Design review of the part built by this model. Coordinates are the model's own, in mm. Face numbers are marked on the shaded views. A direction names the side the tool comes from. Coordinates: 2 decimals unless noted, no trailing zeros. Loops run counter-clockwise (first coordinate to the right, second up) from the corner with the lowest first, then second, coordinate; pieces in that order, holes last. Notation, with made-up numbers: M -40,-8 L 11,-8 A22 cw 11,31 Z; hole C -32.75,82.5 d3. An arc over 180 degrees is marked long. One line per item, written item: value.
```python
from build123d import *

# Parameters (mm, degrees)
F0_W     = 165
F0_H     = 40
F1_DEPTH = 10
F2_SIZE2 = 9.99999
F2_SIZE  = 4.99999
F3_SIZE2 = 4.99999
F3_SIZE  = 9.99999
F4_W     = 44
F4_H     = 4
F5_DEPTH = 18
F4_H_2   = 9
F6_DEPTH = 8


# Not quite as in the source:
# - a fillet or chamfer is up to 0.001 mm smaller than in the source, because OpenCascade refuses the exact size


with BuildPart() as f1:
    # F0 (on Top) → F1 (new body)
    with BuildSketch(Plane.XY):
        with Locations((82.5, 20)):
            Rectangle(F0_W, F0_H)
    extrude(amount=F1_DEPTH)

    # F2 (size 5 and 10 in the source; OpenCascade refuses exactly that, so slightly less here)
    f2_edges = [f1.edges().sort_by_distance(p)[0] for p in [
        (165, 20, 10),
    ]]
    f2_side = f1.faces().sort_by_distance((82.5, 20, 10))[0]
    chamfer(f2_edges, length=F2_SIZE, length2=F2_SIZE2, reference=f2_side)

    # F3 (size 10 and 5 in the source; OpenCascade refuses exactly that, so slightly less here)
    f3_edges = [f1.edges().sort_by_distance(p)[0] for p in [
        (0, 20, 10),
    ]]
    f3_side = f1.faces().sort_by_distance((0, 20, 5))[0]
    chamfer(f3_edges, length=F3_SIZE, length2=F3_SIZE2, reference=f3_side)

    # F4 (on face) → F5 (join)
    with BuildSketch(Plane.XY.offset(10)):
        with Locations((135, 30.5)):
            Rectangle(F4_W, F4_H)
        with Locations((135, 9.5)):
            Rectangle(F4_W, F4_H)
    extrude(amount=F5_DEPTH)

    # F4 (on face) → F6 (join)
    with BuildSketch(Plane.XY.offset(10)):
        with Locations((135, 20)):
            Rectangle(F4_W, F4_H_2)
    extrude(amount=F6_DEPTH)


solid = f1.part
```
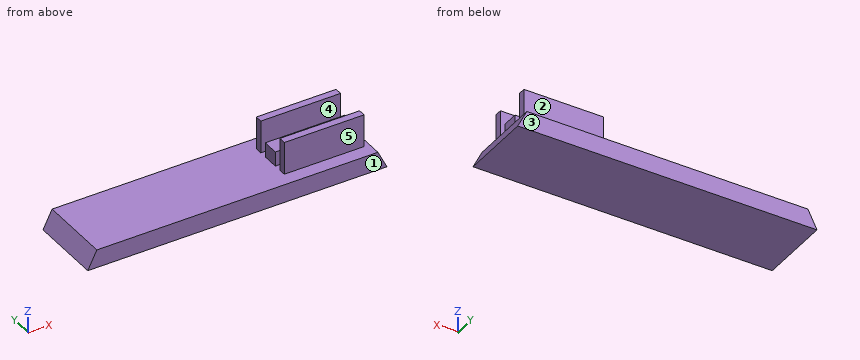
(1) Tool access review of the marked faces 1 and 2: name each direction out of +Z, -Z, +X, -X, +Y, -Y from which nothing blocks a thin tool from reaching the whole face with its end or side.
Reply:
face 1: +Z, -Z, +X, -X, -Y
face 2: +Z, +X, -X, +Y
(2) We need section C-C on x = 116.5. State the section outline as (y, z) points, then the cut area to 3 significant figures.
Reply:
outline: M 0,0 L 40,0 L 40,10 L 32.5,10 L 32.5,28 L 28.5,28 L 28.5,10 L 24.5,10 L 24.5,18 L 15.5,18 L 15.5,10 L 11.5,10 L 11.5,28 L 7.5,28 L 7.5,10 L 0,10 Z
area: 616 mm2
(3) Insertion check: pin 1 (5.5 mm diameter, centred on x = 132.5, z = 17, fed in from -Y); pin 2 (4 mm diameter, centred on y = 6, z = 10, fed in from -X); pin 3 (1.2 mm diameter, centred on y = 30, z = 18.5, fed in from -X); pin 4 (2 mm diameter, centred on x = 125, z = 10.5, fed in from -Y). Each pin has a flat end and moves straight along its axis. Give the tip position at first contact, or say it passes through.
Reply:
pin 1: stops at y = 7.5
pin 2: stops at x = 4
pin 3: stops at x = 113
pin 4: stops at y = 0
(4) To check wall thickness, follow line 1 along Y through (x, z) = (151, 23); line 2 along Z through (x, y) = (43.5, 2); line 3 along X through (y, z) = (30, 16.5). State the ranges of each line that lie inside material, in increasing order. Write a range as [from, to].
Reply:
line 1: y = [7.5, 11.5], [28.5, 32.5]
line 2: z = [0, 10]
line 3: x = [113, 157]
(5) We need section A-A on z = 12.75. State the section outline as (x, y) points.
Reply:
outline: M 113,7.5 L 157,7.5 L 157,11.5 L 113,11.5 Z; M 113,15.5 L 157,15.5 L 157,24.5 L 113,24.5 Z; M 113,28.5 L 157,28.5 L 157,32.5 L 113,32.5 Z
(6) Mouldability with a two-part tool opening along Y and no side actions: class the marked faces 3, 4 and 5 as released by +Y, released by -Y, zero draft, split by the parting line, or undercut.
Reply:
face 3: released by +Y
face 4: undercut
face 5: released by -Y
(7) We need section B-B on z = 24.5. State the section outline as (x, y) points.
Reply:
outline: M 113,7.5 L 157,7.5 L 157,11.5 L 113,11.5 Z; M 113,28.5 L 157,28.5 L 157,32.5 L 113,32.5 Z
